Geometry: final body of the model. Coordinates: model frame, mm. Round coordinates to 2 decimals unless told otherwise and drop trailing zeros. Loops run counter-clockwise (first coordinate to the right, second up) from the corner with the lowest first, then second, coordinate; pieces in that order, holes last. Notation, with made-up numbers: (52.25, 18) - (72.25, 18) arc R21 cw to (72.25, 32) - close; hole circle Ø8 at (81.25, 0). An arc over 180 degrees is marked (long way). Write item = value, one per line. Start each with the question number.
Item 1: Section A-A (x = -67.1). Return loops of the section in (y, z) (3 decimals).
Item 2: First-contact query: pin 1 (4 mm diameter, centred on x = 60, z = -47.5, fed in from -Y). Flat tip, straight axial feed; report the tip coordinate or a pass-through.
Item 3: Line query: line 1 (Z direction, x = 67.1, y = 2.45) (3 decimals). Output: solid intervals per line, ascending. Write a range as from..to.
Item 4: Draft query along X for faces 1 (the flat face through (-79, 3, 1)), 2 (the cylindrical face through (68.353, 2.194, -62.274)), 3 (the flat face through (-1, 5.9, -1)), 4 (the flat face through (79, 3, 1)). Return one class per face: pulls with the +X half, pulls with the -X half, needs draft (parallel to the pull), parting line crosses it, or undercut.
from build123d import *

# Parameters (mm, degrees)
SKETCH1_W                                       = 158
SKETCH1_H                                       = 134.25
BOSS_EXTRUDE1_DEPTH                             = 5.9
CSK_FOR_M3_FLAT_HEAD_MACHINE_SCREW1_D           = 3.4
CSK_FOR_M3_FLAT_HEAD_MACHINE_SCREW1_DEPTH       = 10
CSK_FOR_M3_FLAT_HEAD_MACHINE_SCREW1_CSINK_D     = 6.3
CSK_FOR_M3_FLAT_HEAD_MACHINE_SCREW1_CSINK_ANGLE = 90
CSK_FOR_M3_FLAT_HEAD_MACHINE_SCREW1_TIP         = 1.021463052


with BuildPart() as part:
    # Sketch1 → Boss-Extrude1 (new body)
    with BuildSketch(Plane(origin=(0, 0, 0), x_dir=(1, 0, 0), z_dir=(0, 1, 0))):
        Rectangle(SKETCH1_W, SKETCH1_H)
    extrude(amount=BOSS_EXTRUDE1_DEPTH)

    # CSK for M3 Flat Head Machine Screw1
    with Locations(Plane(origin=(0, 5.9, 0), x_dir=(1, 0, 0), z_dir=(0, 1, 0))):
        with Locations((-67.1, 61.125), (67.1, 61.125)):
            CounterSinkHole(CSK_FOR_M3_FLAT_HEAD_MACHINE_SCREW1_D / 2, CSK_FOR_M3_FLAT_HEAD_MACHINE_SCREW1_CSINK_D / 2, depth=CSK_FOR_M3_FLAT_HEAD_MACHINE_SCREW1_DEPTH, counter_sink_angle=CSK_FOR_M3_FLAT_HEAD_MACHINE_SCREW1_CSINK_ANGLE)
            with Locations((0, 0, -(CSK_FOR_M3_FLAT_HEAD_MACHINE_SCREW1_DEPTH + CSK_FOR_M3_FLAT_HEAD_MACHINE_SCREW1_TIP / 2))):  # 118° drill point
                Cone(0, CSK_FOR_M3_FLAT_HEAD_MACHINE_SCREW1_D / 2, CSK_FOR_M3_FLAT_HEAD_MACHINE_SCREW1_TIP, mode=Mode.SUBTRACT)


solid = part.part
Taken from the geometry:
q1.outline = (0, -67.125) - (5.9, -67.125) - (5.9, -64.275) - (4.45, -62.825) - (0, -62.825) - close; (0, -59.425) - (4.45, -59.425) - (5.9, -57.975) - (5.9, 67.125) - (0, 67.125) - close
q2.pin_1 = 0
q3.line_1 = -67.125..-62.825, -59.425..67.125
q4.face_1 = pulls with the -X half
q4.face_2 = undercut
q4.face_3 = needs draft
q4.face_4 = pulls with the +X half
